```python
from build123d import *

# Parameters (mm, degrees)
SKETCH003_W             = 200
SKETCH003_H             = 200
PAD002_DEPTH            = 100
SKETCH004_W             = 180
SKETCH004_H             = 180
POCKET001_DEPTH         = 90
SKETCH005_R             = 2.5
PAD003_DEPTH            = 50
LINEARPATTERN001_COUNT  = 2
LINEARPATTERN001_PITCH  = 100
BODY003_PLACEMENT_ANGLE = 180


with BuildPart() as part:
    # Sketch003 → Pad002 (new body)
    with BuildSketch(Plane.XY):
        Rectangle(SKETCH003_W, SKETCH003_H)
    extrude(amount=PAD002_DEPTH)

    # Sketch004 (on Face6 of Pad002) → Pocket001 (cut)
    with BuildSketch(Plane.XY.offset(100)):
        Rectangle(SKETCH004_W, SKETCH004_H)
    extrude(amount=-POCKET001_DEPTH, mode=Mode.SUBTRACT)

    # Sketch005 (on Face6 of Pocket001) → Pad003 (join)
    with BuildSketch(Plane.XZ.offset(100)):
        with BuildLine():
            ThreePointArc((-101.243422, 100.055887), (-107.925827, 104.903535), (-110.016374, 96.917056))
            Line((-110.016374, 96.917056), (-99.591536, 85.891823))
            Line((-99.591536, 85.891823), (-99.5, 100.055887))
            Line((-99.5, 100.055887), (-101.243422, 100.055887))
        make_face()
        with Locations((-106.241464, 100.195784)):
            Circle(SKETCH005_R, mode=Mode.SUBTRACT)
    pad003 = extrude(amount=-PAD003_DEPTH)

    # LinearPattern001: Pad003 ×2
    with Locations(*[(0, i * LINEARPATTERN001_PITCH, 0) for i in range(1, LINEARPATTERN001_COUNT)]):
        add(pad003)


with BuildPart() as part_1:
    # Body003 placement: moved
    add(part.part.moved(Location((0, 0, 200.5))).rotate(Axis((0, 0, 200.5), (1, 0, 0)), BODY003_PLACEMENT_ANGLE))


solid = part_1.part
```
The listing builds one solid part. Answer for the finished solid, in the listing's coordinates (mm). A direction names the side the tool comes from. Coordinates: 2 decimals unless noted, no trailing zeros. Loops run counter-clockwise (first coordinate to the right, second up) from the corner with the lowest first, then second, coordinate; pieces in that order, holes last. Notation, with made-up numbers: (87, 2.5) -> (110, 2.5) arc R4 cw to (110, 8.5) -> close; hole circle Ø8 at (-4, 71). An arc over 180 degrees is marked (long way). Return JSON: item names as keys, results as strings. Group by question number.
(1) Determine the mould class of faces 1 (the flat face through (-1, -100, 151)), 2 (the flat face through (-7, 100, 147)), 3 (the flat face through (-1, 90, 145)) for opening direction Y: released by +Y, released by -Y, zero draft, split by the parting line, or undercut.
(2) A cutting plane is placed at A-A on z = 182.5. Write down the section's boundary in (x, y).
(3) Find the intervals of material crossed by probe 1 along X at (y, z) = (57, 129.5); probe 2 along Z at (x, y) = (65.5, 22.5), in increasing order. Write a range as from..to.
(4) Which of the six approach directions +Z, -Z, +X, -X, +Y, -Y give full straight-line access (tool end or side, diameter ignored) to faces 4 (the flat face through (-105.078, -24.65, 108.805)), 5 (the flat face through (-104, 50, 105)), 6 (the flat face through (90, 1, 145)), 7 (the flat face through (-8, 96, 100.5))?
(5) Given pin 1 Ø0.5 at (x, y) = (-100.5, 79) entering from -Z; pin 2 Ø9.5 at (x, z) = (-107.5, 106.5) entering from -Y; pin 3 Ø5 at (y, z) = (49.5, 158.5) entering from -X, each flat-ended and moving along its own axis, determine where each tip first touches the part or whether it passes through.
(6) A cutting plane is placed at D-D on y = 68.5. Write down the section's boundary in (x, z).
(7) A cutting plane is placed at B-B on y = 25.5. Write down the section's boundary in (x, z), and give its area (3 significant figures).
The answers:
{
 "1": {"face 1": "released by -Y", "face 2": "released by +Y", "face 3": "undercut"},
 "2": {"outline": "(-100, -100) -> (100, -100) -> (100, 100) -> (-100, 100) -> close; hole (-90, -90) -> (90, -90) -> (90, 90) -> (-90, 90) -> close"},
 "3": {"probe 1": "x = -100..-90, 90..100", "probe 2": "z = 190.5..200.5"},
 "4": {"face 4": "+Z, -X, +Y, -Y", "face 5": "+Z, -Z, -X", "face 6": "-Z", "face 7": "-Z, +X, +Y, -Y"},
 "5": {"pin 1": "stops at z = 100.44", "pin 2": "stops at y = -50", "pin 3": "stops at x = -100"},
 "6": {"outline": "(-110.02, 103.58) arc R5 ccw (long way) to (-101.24, 100.44) -> (-99.5, 100.44) -> (-99.5, 100.5) -> (-90, 100.5) -> (-90, 190.5) -> (90, 190.5) -> (90, 100.5) -> (100, 100.5) -> (100, 200.5) -> (-100, 200.5) -> (-100, 114.18) -> close; hole circle Ø5 at (-106.24, 100.3)"},
 "7": {"outline": "(-100, 100.5) -> (-90, 100.5) -> (-90, 190.5) -> (90, 190.5) -> (90, 100.5) -> (100, 100.5) -> (100, 200.5) -> (-100, 200.5) -> close", "area": "3,800 mm^2"}
}
